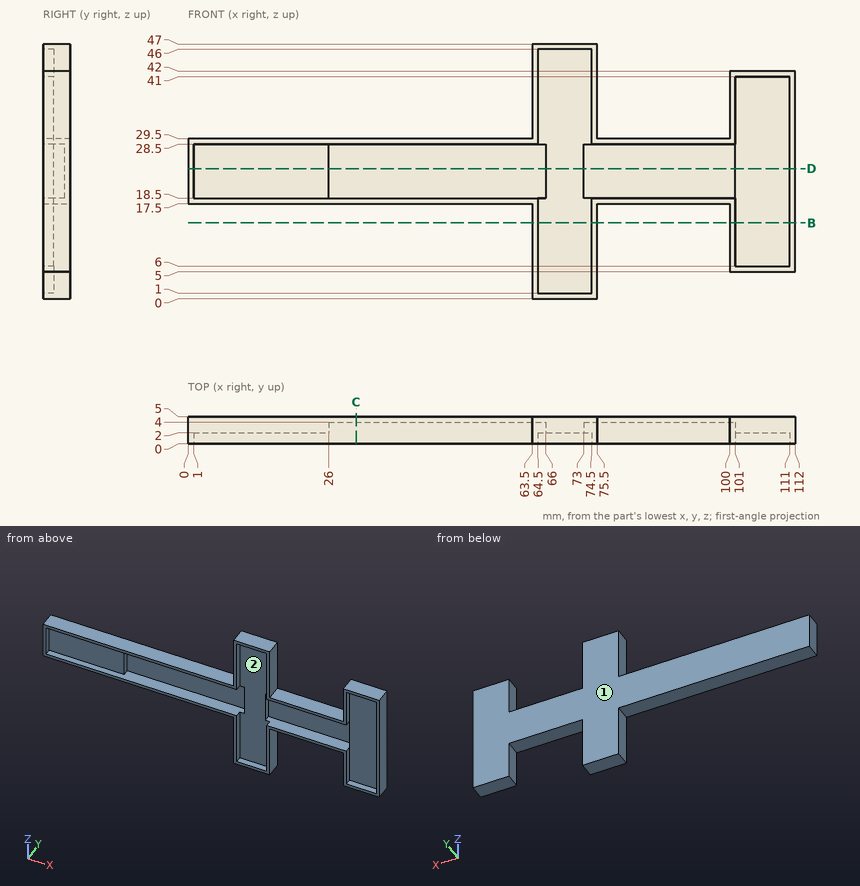
Input: dimensioned drawing with shaded views. Units: mm. Origin: part minimum x, y, z. Round coordinates to 2 decimals unless told otherwise and drop trailing zeros. Order: outer loops, then holes, each group sorted by start corner. A loop starts at its lowest first (then second) coordinate and runs counter-clockwise, first axis right, second up.
Q1. Material intervals for probe 1 along X at (y, z) = (1.4, 32.5); probe 2 along X at (y, z) = (4.1, 30.5); probe 3 along Z at (x, y) = (102.5, 0.4), sorted ascending.
Result sheet:
probe 1: x = 63.5 to 64.5, 74.5 to 75.5, 100 to 101, 111 to 112
probe 2: x = 63.5 to 75.5, 100 to 112
probe 3: z = 5 to 6, 41 to 42
Q2. Pin query (flat end, axial travel): pin 1 (1.5 mm diameter, centred on y = 3.5, z = 13, fed in from -X); pin 2 (2 mm diameter, centred on x = 89, y = 2, fed in from -Z); pin 3 (2 mm diameter, centred on x = 105.5, y = 1, fed in from +Z). Return the tip coordinate at first contact, or that it passes through.
Result sheet:
pin 1: stops at x = 63.5
pin 2: stops at z = 17.5
pin 3: stops at z = 42
Q3. Mould query, pull axis Z, two halves, no side actions, for the marked faces 1 and 2. Classes: released by +Z, released by -Z, zero draft, split by the parting line, or undercut.
Result sheet:
face 1: zero draft
face 2: undercut
Q4. Section D-D, the plane z = 24. Output: boundary loops of the cut face in (x, y).
Result sheet:
outline: (0, 0) - (1, 0) - (1, 2) - (26, 2) - (26, 4) - (66, 4) - (66, 2) - (73, 2) - (73, 4) - (101, 4) - (101, 2) - (111, 2) - (111, 0) - (112, 0) - (112, 5) - (0, 5) - close
Q5. Section C-C, the plane x = 31. Output: boundary loops of the cut face in (y, z).
Result sheet:
outline: (0, 17.5) - (5, 17.5) - (5, 29.5) - (0, 29.5) - (0, 28.5) - (4, 28.5) - (4, 18.5) - (0, 18.5) - close
Q6. Section B-B, the plane z = 14. Output: boundary loops of the cut face in (x, y), and give its area (3 significant figures).
Result sheet:
outline: (63.5, 0) - (64.5, 0) - (64.5, 2) - (74.5, 2) - (74.5, 0) - (75.5, 0) - (75.5, 5) - (63.5, 5) - close; (100, 0) - (101, 0) - (101, 2) - (111, 2) - (111, 0) - (112, 0) - (112, 5) - (100, 5) - close
area: 80.0 mm2
